Design review of the part built by this model. Coordinates are the model's own, in mm. A direction names the side the tool comes from. Coordinates: 2 decimals unless noted, no trailing zeros. Loops run counter-clockwise (first coordinate to the right, second up) from the corner with the lowest first, then second, coordinate; pieces in that order, holes last. Notation, with made-up numbers: (80, 20) -> (84, 20) arc R24 ccw to (84, 48) -> close; hole circle Ø8 at (50, 42.5). An arc over 180 degrees is marked (long way). Answer as a JSON object with one key per item and string values.
```python
from build123d import *

# Parameters (mm, degrees)
F1_DEPTH = 63.5
F0_W     = 27.987413
F0_H     = 19.05
F2_DEPTH = 25.4
F3_DEPTH = 7.9375
F5_R     = 6.35


with BuildPart() as f1:
    # F0 (on Front) → F1 (new body, symmetric)
    with BuildSketch(Plane.XZ):
        Polygon((22.225, 9.525), (-41.275, 9.525), (-41.275, -9.525), (41.275, -9.525), (41.275, 9.525), align=None)
    extrude(amount=F1_DEPTH, both=True)

    # F0 (on Front) → F2 (join, symmetric)
    with BuildSketch(Plane.XZ):
        with BuildLine():
            Line((22.225, 27.0002), (22.225, 9.525))
            Line((22.225, 9.525), (41.275, 9.525))
            Line((41.275, 9.525), (41.275, 27.0002))
            ThreePointArc((41.275, 27.0002), (45.92468, 38.22552), (57.15, 42.8752))
            Line((57.15, 42.8752), (60.325, 42.8752))
            Line((60.325, 42.8752), (60.325, 61.9252))
            Line((60.325, 61.9252), (57.15, 61.9252))
            ThreePointArc((57.15, 61.9252), (32.454296, 51.695904), (22.225, 27.0002))
        make_face()
        with Locations((74.318706, 52.4002)):
            Rectangle(F0_W, F0_H)
    extrude(amount=F2_DEPTH, both=True)

    # F0 (on Front) → F3 (join, symmetric)
    with BuildSketch(Plane.XZ):
        with BuildLine():
            add(Edge.make_bspline(
                [(-41.275, 9.525), (-38.495697, 38.790718), (40.304676, 71.696699), (60.325, 61.9252)],
                knots=[0, 0, 0, 0, 114.316845, 114.316845, 114.316845, 114.316845], degree=3))
            Line((-41.275, 9.525), (22.225, 9.525))
            Line((22.225, 9.525), (22.225, 27.0002))
            ThreePointArc((22.225, 27.0002), (32.454296, 51.695904), (57.15, 61.9252))
            Line((57.15, 61.9252), (60.325, 61.9252))
        make_face()
    extrude(amount=F3_DEPTH, both=True)

    # F0 (on Front) → F4 (revolve)
    with BuildSketch(Plane.XZ):
        Polygon((88.312413, 66.675), (88.312413, 61.9252), (88.312413, 42.8752), (88.312413, 38.1), (111.125, 38.1), (111.125, 66.675), align=None)
    revolve(axis=Axis((88.312413, 0, 54.7751), (0, 0, 1)))

    # F5
    f5_edges = [f1.edges().sort_by_distance(p)[0] for p in [
        (-41.275, -63.5, 0),
        (41.275, -63.5, 0),
        (-41.275, 63.5, 0),
        (41.275, 63.5, 0),
    ]]
    fillet(f5_edges, radius=F5_R)


solid = f1.part
```
1) Clearance check with flat-ended pins moving along their axes: pin 1 Ø8.5 at (y, z) = (18.5, 15.5) entering from -X (3 decimals); pin 2 Ø16.5 at (x, y) = (-20, 35) entering from +Z (3 decimals); pin 3 Ø10 at (x, z) = (48, 43.5) entering from -Y. State where each tip first meets the part, or that it passes through.
Completed:
{"pin 1": "x = 22.225", "pin 2": "z = 9.525", "pin 3": "y = -25.4"}
2) Add section B-B, the plane x = 98. Give the boundary of the cut face in (y, z) (3 decimals), and give its area (3 significant figures).
Completed:
{"outline": "(-20.653, 38.1) -> (20.653, 38.1) -> (20.653, 66.675) -> (-20.653, 66.675) -> close", "area": "1,180 mm²"}
3) For faces 1 (the flat face through (47, 25.4, 42)), 2 (the flat face through (89, 0, 38.1)), 3 (the flat face through (66, -6, 61.925)), 4 (the cylindrical face through (32.73, -16.79, 51.97)), 5 (the flat face through (47, -25.4, 42)), list the 3-axis set-ups (+Z, -Z, +X, -X, +Y, -Y) from which the entire face can be reached by the end or side of a thin tool; tool diameter is ignored.
Completed:
{"face 1": "+Z, +X, -X, +Y", "face 2": "-Z, +X, +Y, -Y", "face 3": "+Z", "face 4": "+Z, -X, -Y", "face 5": "+Z, +X, -X, -Y"}
4) Add section C-C, the plane y = 38.5. Give the boundary of the cut face in (x, z) (3 decimals), and give its area (3 significant figures).
Completed:
{"outline": "(-41.275, -9.525) -> (41.275, -9.525) -> (41.275, 9.525) -> (-41.275, 9.525) -> close", "area": "1,570 mm²"}
5) Wall thickness on probe 1 along Y at (x, z) = (35, 6.5); probe 2 along Y at (x, z) = (0, 19.5); probe 3 along Z at (x, y) = (39, -40.5) (3 decimals): over which ranges is each line inside the solid? List them lowest first.
Completed:
{"probe 1": "-63.5 to 63.5", "probe 2": "-7.94 to 7.94", "probe 3": "-9.525 to 9.525"}
6) Add section A-A, the plane y = 21. Give the boundary of the cut face in (x, z) (3 decimals).
Completed:
{"outline": "(-41.275, -9.525) -> (41.275, -9.525) -> (41.275, 27) arc R15.875 cw to (57.15, 42.875) -> (79.401, 42.875) -> (79.401, 38.1) -> (97.224, 38.1) -> (97.224, 66.675) -> (79.401, 66.675) -> (79.401, 61.925) -> (57.15, 61.925) arc R34.925 ccw to (22.225, 27) -> (22.225, 9.525) -> (-41.275, 9.525) -> close"}
